from build123d import *

# Parameters (mm, degrees)
MODEL_R                         = 1.7
MODEL_R_2                       = 11.05
MODEL_R_3                       = 2.7
AUFSATZ_LINEAR_AUSTRAGEN1_DEPTH = 3


with BuildPart() as part:
    # Model → Aufsatz-Linear austragen1 (new body)
    with BuildSketch(Plane.XY):
        with BuildLine():
            Line((19, 10.923593129), (19, 3))
            ThreePointArc((19, 3), (19.878679656, 0.878679656), (22, 0))
            Line((22, 0), (58, 0))
            ThreePointArc((58, 0), (60.121320344, 0.878679656), (61, 3))
            Line((61, 3), (61, 10.923593129))
            Line((61, 10.923593129), (77.915065607, 27.838658665))
            ThreePointArc((77.915065607, 27.838658665), (79.783724343, 32.349999929), (77.915065607, 36.861341193))
            Line((77.915065607, 36.861341193), (44.511341215, 70.265065599))
            ThreePointArc((44.511341215, 70.265065599), (39.999999949, 72.133724339), (35.488658682, 70.265065603))
            Line((35.488658682, 70.265065603), (2.084934387, 36.861341261))
            ThreePointArc((2.084934387, 36.861341261), (0.216275654, 32.349999998), (2.08493439, 27.838658736))
            Line((2.08493439, 27.838658736), (19, 10.923593129))
        make_face()
        with Locations((40, 10.429689783)):
            Circle(MODEL_R, mode=Mode.SUBTRACT)
        with Locations((61.920310217, 32.35)):
            Circle(MODEL_R, mode=Mode.SUBTRACT)
        with Locations((40, 54.270310217)):
            Circle(MODEL_R, mode=Mode.SUBTRACT)
        with Locations((18.079689783, 32.35)):
            Circle(MODEL_R, mode=Mode.SUBTRACT)
        with Locations((40, 32.35)):
            Circle(MODEL_R_2, mode=Mode.SUBTRACT)
        with Locations((73.4, 32.35)):
            Circle(MODEL_R_3, mode=Mode.SUBTRACT)
        with Locations((40, 65.75)):
            Circle(MODEL_R_3, mode=Mode.SUBTRACT)
        with Locations((6.6, 32.35)):
            Circle(MODEL_R_3, mode=Mode.SUBTRACT)
        with BuildLine():
            Line((32.7, 10), (32.7, 17.5))
            ThreePointArc((32.7, 17.5), (30, 20.2), (27.3, 17.5))
            Line((27.3, 17.5), (27.3, 10))
            ThreePointArc((27.3, 10), (30, 7.3), (32.7, 10))
        make_face(mode=Mode.SUBTRACT)
        with BuildLine():
            Line((47.3, 10), (47.3, 17.5))
            ThreePointArc((47.3, 17.5), (50, 20.2), (52.7, 17.5))
            Line((52.7, 17.5), (52.7, 10))
            ThreePointArc((52.7, 10), (50, 7.3), (47.3, 10))
        make_face(mode=Mode.SUBTRACT)
    extrude(amount=AUFSATZ_LINEAR_AUSTRAGEN1_DEPTH)


solid = part.part
The model under review builds one solid part; all positions refer to its coordinate system, in mm. A direction names the side the tool comes from. Give positions to 0.01 mm unless a question says otherwise; leave off trailing zeros. Order: outer loops, then holes, each group sorted by start corner. A loop starts at its lowest first (then second) coordinate and runs counter-clockwise, first axis right, second up. Notation, with made-up numbers: M 25,79 L 67,79 A20 cw 67,99 Z; hole C 36,27.5 d5. An arc over 180 degrees is marked long. Answer in a Markdown table with one row per item. Add a question column.
1. Add section C-C on y = 65.75. State the section outline as (x, z) points.
2. Machinability: for faces 1 (the flat face through (19, 7, 1)), 2 (the flat face through (61, 7, 1)), 3 (the cylindrical face through (29.9, 7.3, 1.5)), which of the approach directions +Z, -Z, +X, -X, +Y, -Y give a long, thin tool a straight path to every point of the face, cutting with its end or side? Answer none if there is none.
3. Mouldability with a two-part tool opening along X and no side actions: class faces 4 (the flat face through (61.447, 53.329, 1.479)), 5 (the cylindrical face through (0.217, 32.42, 1.479)), 6 (the cylindrical face through (6.015, 29.714, 1.479)) as released by +X, released by -X, zero draft, split by the parting line, or undercut.
4. Add section B-B on y = 32.35. State the section outline as (x, z) points, plus the area to 3 significant figures.
5. Add section A-A on x = 40. State the section outline as (y, z) points.
6. Add section D-D on x = 73. State the section outline as (y, z) points.
7. For pin 1 Ø1 at (x, z) = (70.5, 1.5) entering from -Y, flat-tipped, find the tip position at first contact; note if it passes through.
8. To check wall thickness, follow line 1 along Y through (x, z) = (40, 2.4); line 2 along Y through (x, z) = (39, 1.55); line 3 along X through (y, z) = (19.5, 0.95). State the ranges of each line that lie inside material, in increasing order.
The answers:
| question | item | result |
|---|---|---|
| 1 | outline | M 30.97,0 L 37.3,0 L 37.3,3 L 30.97,3 Z; M 42.7,0 L 49.03,0 L 49.03,3 L 42.7,3 Z |
| 2 | face 1 | +Z, -Z, -X, -Y |
| 2 | face 2 | +Z, -Z, +X, -Y |
| 2 | face 3 | +Z, -Z |
| 3 | face 4 | released by +X |
| 3 | face 5 | released by -X |
| 3 | face 6 | undercut |
| 4 | outline | M 0.22,0 L 3.9,0 L 3.9,3 L 0.22,3 Z; M 9.3,0 L 16.38,0 L 16.38,3 L 9.3,3 Z; M 19.78,0 L 28.95,0 L 28.95,3 L 19.78,3 Z; M 51.05,0 L 60.22,0 L 60.22,3 L 51.05,3 Z; M 63.62,0 L 70.7,0 L 70.7,3 L 63.62,3 Z; M 76.1,0 L 79.78,0 L 79.78,3 L 76.1,3 Z |
| 4 | area | 120 mm2 |
| 5 | outline | M 0,0 L 8.73,0 L 8.73,3 L 0,3 Z; M 12.13,0 L 21.3,0 L 21.3,3 L 12.13,3 Z; M 43.4,0 L 52.57,0 L 52.57,3 L 43.4,3 Z; M 55.97,0 L 63.05,0 L 63.05,3 L 55.97,3 Z; M 68.45,0 L 72.13,0 L 72.13,3 L 68.45,3 Z |
| 6 | outline | M 22.92,0 L 29.68,0 L 29.68,3 L 22.92,3 Z; M 35.02,0 L 41.78,0 L 41.78,3 L 35.02,3 Z |
| 7 | pin 1 | y = 19.92 |
| 8 | line 1 | 0 to 8.73, 12.13 to 21.3, 43.4 to 52.57, 55.97 to 63.05, 68.45 to 72.13 |
| 8 | line 2 | 0 to 9.05, 11.8 to 21.35, 43.35 to 52.9, 55.65 to 63.24, 68.26 to 72.05 |
| 8 | line 3 | 10.42 to 28.19, 31.81 to 48.19, 51.81 to 69.58 |
